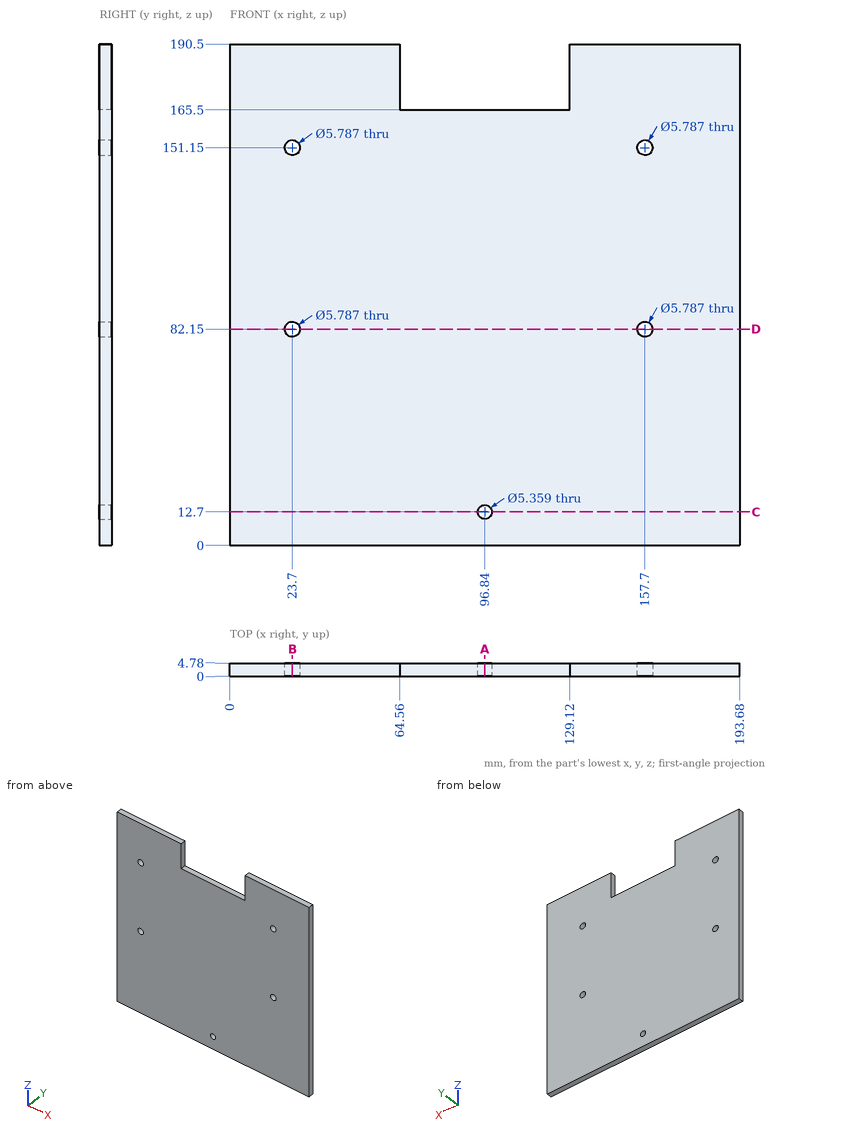
Study the drawing (mm; zero at the part's minimum x, y, z) and answer. Coordinates: 2 decimals unless noted, no trailing zeros. Loops run counter-clockwise (first coordinate to the right, second up) from the corner with the lowest first, then second, coordinate; pieces in that order, holes last. Notation, with made-up numbers: (-2, -31.75) -> (2, -31.75) arc R22 ccw to (2, -0.75) -> close; hole circle Ø7 at (-20, 19.25). An arc over 180 degrees is marked (long way). Answer as CSV lines item,"result".
1) A flat-ended cylindrical pin translates along its axis: pin 1 (3 mm diameter, centred on x = 96.84, z = 12.7, fed in from +Y). Find the tip coordinate at first contact, or state that the pin passes through.
A:
pin 1,"passes through"
2) The part is cut by section B-B (x = 23.7). Give the vertices of the cut face in (y, z).
A:
outline,"(0, 0) -> (4.78, 0) -> (4.78, 79.26) -> (0, 79.26) -> close; (0, 85.04) -> (4.78, 85.04) -> (4.78, 148.26) -> (0, 148.26) -> close; (0, 154.04) -> (4.78, 154.04) -> (4.78, 190.5) -> (0, 190.5) -> close"
3) The part is cut by section C-C (z = 12.7). Give the vertices of the cut face in (x, y), and give its area (3 significant figures).
A:
outline,"(0, 0) -> (94.16, 0) -> (94.16, 4.78) -> (0, 4.78) -> close; (99.52, 0) -> (193.68, 0) -> (193.68, 4.78) -> (99.52, 4.78) -> close"
area,"900 mm²"
4) The part is cut by section D-D (z = 82.15). Give the vertices of the cut face in (x, y).
A:
outline,"(0, 0) -> (20.81, 0) -> (20.81, 4.78) -> (0, 4.78) -> close; (26.59, 0) -> (154.81, 0) -> (154.81, 4.78) -> (26.59, 4.78) -> close; (160.59, 0) -> (193.68, 0) -> (193.68, 4.78) -> (160.59, 4.78) -> close"
5) Straight lines are drawn through the part: probe 1 along Z at (x, y) = (157.7, 3.85); probe 2 along X at (y, z) = (1, 82.15); probe 3 along X at (y, z) = (0.65, 183.5). For each, find the intervals that lie inside material, in ascending order.
A:
probe 1,"z = 0 to 79.26, 85.04 to 148.26, 154.04 to 190.5"
probe 2,"x = 0 to 20.81, 26.59 to 154.81, 160.59 to 193.68"
probe 3,"x = 0 to 64.56, 129.12 to 193.68"
6) The part is cut by section A-A (x = 96.84). Give the vertices of the cut face in (y, z).
A:
outline,"(0, 0) -> (4.78, 0) -> (4.78, 10.02) -> (0, 10.02) -> close; (0, 15.38) -> (4.78, 15.38) -> (4.78, 165.5) -> (0, 165.5) -> close"
